For this review, take the finished solid that the model builds, in its own axes (mm). Face numbers are marked on the shaded views. A direction names the side the tool comes from. Round coordinates to 2 decimals unless told otherwise and drop trailing zeros. Loops run counter-clockwise (first coordinate to the right, second up) from the corner with the lowest first, then second, coordinate; pieces in that order, holes last. Notation, with made-up numbers: M 42,72.5 L 76,72.5 A14 ccw 76,91.5 Z; hole C -35.5,72 d6. An arc over 180 degrees is marked long. One line per question, with ' | ' between items. Start each with the question number.
1) We need section B-B (y = -13.75). Give the boundary of the cut face in (x, z).
2) We need section C-C (z = 0). Give the boundary of the cut face in (x, y), and give its area (3 significant figures).
3) We need section D-D (x = -19). Give the boundary of the cut face in (y, z).
4) We need section A-A (x = 10.5). Give the boundary of the cut face in (y, z).
5) Mouldability with a two-part tool opening along X and no side actions: class the marked faces 1, 2 and 3 as pulls with the +X half, pulls with the -X half, needs draft (parallel to the pull), parting line crosses it, or undercut.
6) For probe 1 along X at (y, z) = (2.35, -32.5); probe 2 along Z at (x, y) = (46, 2.25); probe 3 along Z at (x, y) = (23, 1.95), list the stretches that pass through material, from the lowest coordinate up. Write a range as from..to.
7) For the marked faces 4, 5 and 6, list the 3-axis set-ups (+Z, -Z, +X, -X, +Y, -Y) from which the entire face can be reached by the end or side of a thin tool; tool diameter is ignored.
8) For pin 1 Ø4 at (x, z) = (20, 25.5) entering from -Y; pin 2 Ø6 at (y, z) = (-2.5, 17.5) entering from +X; pin 3 Ø4 at (x, z) = (-53.5, 6) entering from +Y; pin 4 Ø3 at (x, y) = (-11, 2.5) entering from -Z, all flat-tipped, find the tip position at first contact; note any pin that passes through.
```python
from build123d import *

# Parameters (mm, degrees)
TABLE_DEPTH                  = 4
PIEDS_START                  = 17
PIEDS_DEPTH                  = 17
ENL_V_MAT_EXTRU_3_DEPTH      = 93.240175629
ENL_V_MAT_EXTRU_3_DEPTH_BACK = 93.240175629
ESQUISSE5_W                  = 5
ESQUISSE5_H                  = 18
ENL_V_MAT_EXTRU_4_DEPTH      = 93.240175629
ENL_V_MAT_EXTRU_4_DEPTH_BACK = 93.240175629
ESQUISSE6_W                  = 43
ESQUISSE6_H                  = 18
CONG_1_R                     = 10
CHANFREIN1_SIZE              = 1
CONG_2_R                     = 3
ESQUISSE3_R                  = 1
ENL_V_MAT_EXTRU_5_DEPTH      = 18
ENL_V_MAT_EXTRU_6_DEPTH      = 93.240175629
ENL_V_MAT_EXTRU_6_DEPTH_BACK = 93.240175629
ESQUISSE4_R                  = 1
ESQUISSE8_W                  = 58
ESQUISSE8_H                  = 72
ENL_V_MAT_EXTRU_7_DEPTH      = 1
ENL_V_MAT_EXTRU_8_DEPTH      = 1
ENL_V_MAT_EXTRU_9_DEPTH      = 93.240175629
ENL_V_MAT_EXTRU_9_DEPTH_BACK = 93.240175629
ESQUISSE11_W                 = 53
ESQUISSE11_H                 = 1
CONG_3_R                     = 1
CONG_4_R                     = 3


with BuildPart() as part:
    # Esquisse1 → table (new body)
    with BuildSketch(Plane(origin=(0, 0, 0), x_dir=(1, 0, 0), z_dir=(0, 1, 0))):
        with BuildLine():
            Line((-49, -57.5), (49, -57.5))
            ThreePointArc((49, -57.5), (63.142135624, -51.642135624), (69, -37.5))
            Line((69, -37.5), (69, 37.5))
            ThreePointArc((69, 37.5), (63.142135624, 51.642135624), (49, 57.5))
            Line((49, 57.5), (-49, 57.5))
            ThreePointArc((-49, 57.5), (-63.142135624, 51.642135624), (-69, 37.5))
            Line((-69, 37.5), (-69, -37.5))
            ThreePointArc((-69, -37.5), (-63.142135624, -51.642135624), (-49, -57.5))
        make_face()
    extrude(amount=TABLE_DEPTH)

    # Esquisse2 → pieds (add)
    with BuildSketch(Plane.XZ.offset(PIEDS_START)):
        with BuildLine():
            Line((-49, 57.5), (-49, 37.5))
            Line((-49, 37.5), (-69, 37.5))
            ThreePointArc((-69, 37.5), (-63.142135624, 51.642135624), (-49, 57.5))
        make_face()
        with BuildLine():
            Line((-69, -37.5), (-49, -37.5))
            Line((-49, -37.5), (-49, -57.5))
            ThreePointArc((-49, -57.5), (-63.142135624, -51.642135624), (-69, -37.5))
        make_face()
        with BuildLine():
            Line((49, -57.5), (49, -37.5))
            Line((49, -37.5), (69, -37.5))
            ThreePointArc((69, -37.5), (63.142135624, -51.642135624), (49, -57.5))
        make_face()
        with BuildLine():
            Line((49, 57.5), (49, 37.5))
            Line((49, 37.5), (69, 37.5))
            ThreePointArc((69, 37.5), (63.142135624, 51.642135624), (49, 57.5))
        make_face()
    extrude(amount=-PIEDS_DEPTH)

    # Esquisse5 → Enlèv. mat.-Extru.3 (cut, two sides: drawn at the far end of the back side and taken through both)
    with BuildSketch(Plane(origin=(0, 4, 0), x_dir=(1, 0, 0), z_dir=(0, 1, 0)).offset(-ENL_V_MAT_EXTRU_3_DEPTH_BACK)):
        with Locations((-26.5, 48.5)):
            Rectangle(ESQUISSE5_W, ESQUISSE5_H)
        with Locations((21.5, 48.5)):
            Rectangle(ESQUISSE5_W, ESQUISSE5_H)
        with Locations((-26.5, -48.5)):
            Rectangle(ESQUISSE5_W, ESQUISSE5_H)
        with Locations((21.5, -48.5)):
            Rectangle(ESQUISSE5_W, ESQUISSE5_H)
    extrude(amount=ENL_V_MAT_EXTRU_3_DEPTH + ENL_V_MAT_EXTRU_3_DEPTH_BACK, mode=Mode.SUBTRACT)

    # Esquisse6 → Enlèv. mat.-Extru.4 (cut, two sides: drawn at the far end of the back side and taken through both)
    with BuildSketch(Plane(origin=(0, 4, 0), x_dir=(1, 0, 0), z_dir=(0, 1, 0)).offset(-ENL_V_MAT_EXTRU_4_DEPTH_BACK)):
        with Locations((-2.5, 48.5)):
            Rectangle(ESQUISSE6_W, ESQUISSE6_H)
        with Locations((-2.5, -48.5)):
            Rectangle(ESQUISSE6_W, ESQUISSE6_H)
    extrude(amount=ENL_V_MAT_EXTRU_4_DEPTH + ENL_V_MAT_EXTRU_4_DEPTH_BACK, mode=Mode.SUBTRACT)

    # Congé1
    cong_1_edges = [part.edges().sort_by_distance(p)[0] for p in [
        (24, 2, 57.5),
        (-29, 2, -57.5),
        (24, 2, -57.5),
        (-29, 2, 57.5),
    ]]
    fillet(cong_1_edges, radius=CONG_1_R)

    # Chanfrein1
    chanfrein1_edges = [part.edges().sort_by_distance(p)[0] for p in [
        (59, -17, -37.5),
        (49, -17, -47.5),
        (63.142135624, -17, -51.642135624),
        (-49, -17, -47.5),
        (-59, -17, -37.5),
        (-63.142135624, -17, -51.642135624),
        (-59, -17, 37.5),
        (-49, -17, 47.5),
        (-63.142135624, -17, 51.642135624),
        (59, -17, 37.5),
        (63.142135624, -17, 51.642135624),
        (49, -17, 47.5),
    ]]
    chamfer(chanfrein1_edges, length=CHANFREIN1_SIZE)

    # Congé2
    cong_2_edges = [part.edges().sort_by_distance(p)[0] for p in [
        (49, -8, 37.5),
        (49, -8, -37.5),
        (-49, -8, -37.5),
        (-49, -8, 37.5),
    ]]
    fillet(cong_2_edges, radius=CONG_2_R)

    # Esquisse3 → Enlèv. mat.-Extru.5 (cut)
    with BuildSketch(Plane(origin=(0, 4, 0), x_dir=(1, 0, 0), z_dir=(0, 1, 0))):
        with Locations(Location((-10, -32.5, 0), (0, 0, 270))):
            Circle(ESQUISSE3_R)
        with Locations(Location((-61, -32.5, 0), (0, 0, 270))):
            Circle(ESQUISSE3_R)
        with Locations(Location((-61, 32.5, 0), (0, 0, 270))):
            Circle(ESQUISSE3_R)
        with Locations(Location((-10, 32.5, 0), (0, 0, 270))):
            Circle(ESQUISSE3_R)
    extrude(amount=-ENL_V_MAT_EXTRU_5_DEPTH, mode=Mode.SUBTRACT)

    # Esquisse4 → Enlèv. mat.-Extru.6 (cut, two sides: drawn at the far end of the back side and taken through both)
    with BuildSketch(Plane(origin=(0, 4, 0), x_dir=(1, 0, 0), z_dir=(0, 1, 0)).offset(-ENL_V_MAT_EXTRU_6_DEPTH_BACK)):
        with Locations(Location((2, -27, 0), (0, 0, 270))):
            Circle(ESQUISSE4_R)
        with Locations(Location((46, 17, 0), (0, 0, 270))):
            Circle(ESQUISSE4_R)
        with Locations(Location((23, 19, 0), (0, 0, 270))):
            Circle(ESQUISSE4_R)
    extrude(amount=ENL_V_MAT_EXTRU_6_DEPTH + ENL_V_MAT_EXTRU_6_DEPTH_BACK, mode=Mode.SUBTRACT)

    # Esquisse8 → Enlèv. mat.-Extru.7 (cut)
    with BuildSketch(Plane(origin=(0, 4, 0), x_dir=(1, 0, 0), z_dir=(0, 1, 0))):
        with Locations((-35.5, 0)):
            Rectangle(ESQUISSE8_W, ESQUISSE8_H)
    extrude(amount=-ENL_V_MAT_EXTRU_7_DEPTH, mode=Mode.SUBTRACT)

    # Esquisse10 → Enlèv. mat.-Extru.8 (cut)
    with BuildSketch(Plane(origin=(0, 4, 0), x_dir=(1, 0, 0), z_dir=(0, 1, 0))):
        Polygon((-2.5, -31.5), (50.207106781, -31.5), (60.5, -21.207106781), (60.5, 19.207106781), (48.207106781, 31.5), (7.792893219, 31.5), (-2.5, 21.207106781), align=None)
    extrude(amount=-ENL_V_MAT_EXTRU_8_DEPTH, mode=Mode.SUBTRACT)

    # Esquisse11 → Enlèv. mat.-Extru.9 (cut, two sides: drawn at the far end of the back side and taken through both)
    with BuildSketch(Plane(origin=(0, 4, 0), x_dir=(1, 0, 0), z_dir=(0, 1, 0)).offset(-ENL_V_MAT_EXTRU_9_DEPTH_BACK)):
        with Locations((-2.5, 39)):
            Rectangle(ESQUISSE11_W, ESQUISSE11_H)
        with Locations((-2.5, -39)):
            Rectangle(ESQUISSE11_W, ESQUISSE11_H)
    extrude(amount=ENL_V_MAT_EXTRU_9_DEPTH + ENL_V_MAT_EXTRU_9_DEPTH_BACK, mode=Mode.SUBTRACT)

    # Congé3
    cong_3_edges = [part.edges().sort_by_distance(p)[0] for p in [
        (24, 2, -38.5),
        (-29, 2, -38.5),
        (-29, 2, 38.5),
        (24, 2, 38.5),
    ]]
    fillet(cong_3_edges, radius=CONG_3_R)

    # Congé4
    # the kernel refuses this fillet: 3 mm, written as the material it takes off along each edge
    with BuildSketch(Plane(origin=(69, -24.858353806, 37.5), x_dir=(-1, 0, 0), z_dir=(0, 1, 0)), Plane(origin=(-69, -24.858353806, -37.5), x_dir=(1, 0, 0), z_dir=(0, 1, 0)), Plane(origin=(49, -24.858353806, -57.5), x_dir=(0, 0, 1), z_dir=(0, 1, 0)), Plane(origin=(-49, -24.858353806, 57.5), x_dir=(0, 0, -1), z_dir=(0, 1, 0))) as cong_4_piece_1:
        with BuildLine():
            CenterArc((3.266799469, 3), CONG_4_R, 169.835751378, 100.164248622)
            ThreePointArc((0.313881729, 3.529411765), (0.078624979, 1.771670761), (0, 0))
            Line((0, 0), (3.266799469, 0))
        make_face()
    extrude(amount=24.858353806, mode=Mode.SUBTRACT)
    with BuildSketch(Plane(origin=(-49, -24.858353806, -57.5), x_dir=(0, 0, 1), z_dir=(0, 1, 0)), Plane(origin=(-69, -24.858353806, 37.5), x_dir=(1, 0, 0), z_dir=(0, 1, 0)), Plane(origin=(69, -24.858353806, -37.5), x_dir=(-1, 0, 0), z_dir=(0, 1, 0)), Plane(origin=(49, -24.858353806, 57.5), x_dir=(0, 0, -1), z_dir=(0, 1, 0))) as cong_4_piece_2:
        with BuildLine():
            CenterArc((3.266799469, -3), CONG_4_R, 90, 100.164248622)
            ThreePointArc((0.313881729, -3.529411765), (0.078624979, -1.771670761), (0, 0))
            Line((0, 0), (3.266799469, 0))
        make_face()
    extrude(amount=24.858353806, mode=Mode.SUBTRACT)


solid = part.part
```
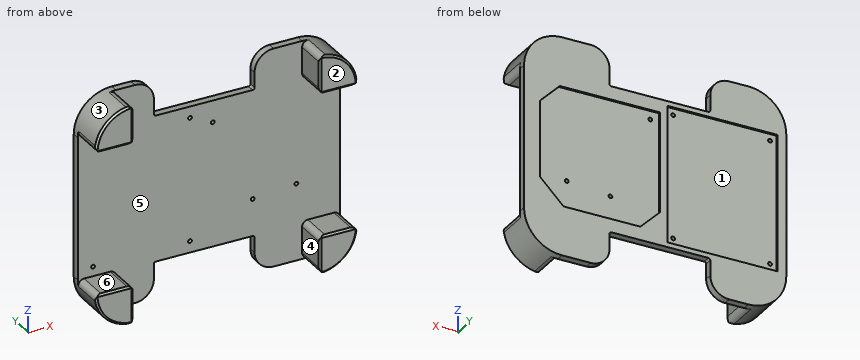
Answers below:
1) outline: M -68.69,-41.03 A20 ccw -52.53,-57.19 A3 ccw -49,-54.23 L -49,-40.5 A3 ccw -52,-37.5 L -65.73,-37.5 A3 ccw Z; M -68.69,41.03 A3 ccw -65.73,37.5 L -52,37.5 A3 ccw -49,40.5 L -49,54.23 A3 ccw -52.53,57.19 A20 ccw Z; M 49,-54.23 A3 ccw 52.53,-57.19 A20 ccw 68.69,-41.03 A3 ccw 65.73,-37.5 L 52,-37.5 A3 ccw 49,-40.5 Z; M 49,40.5 A3 ccw 52,37.5 L 65.73,37.5 A3 ccw 68.69,41.03 A20 ccw 52.53,57.19 A3 ccw 49,54.23 Z
2) outline: M -69,0 L 69,0 L 69,4 L 60.5,4 L 60.5,3 L -2.5,3 L -2.5,4 L -6.5,4 L -6.5,3 L -64.5,3 L -64.5,4 L -69,4 Z | area: 431 mm^2
3) outline: M 0,-38.5 L 4,-38.5 L 4,-36 L 3,-36 L 3,36 L 4,36 L 4,38.5 L 0,38.5 Z
4) outline: M 0,-38.5 L 4,-38.5 L 4,-31.5 L 3,-31.5 L 3,31.5 L 4,31.5 L 4,38.5 L 0,38.5 Z
5) face 1: undercut | face 2: needs draft | face 3: pulls with the -X half
6) probe 1: -69..-62, -60..-11, -9..69 | probe 2: -57.5..-18, -16..57.5 | probe 3: -38.5..-20, -18..38.5
7) face 4: +Z, -Z, -Y | face 5: -Y | face 6: +X, -X, -Y
8) pin 1: y = 0 | pin 2: x = 69 | pin 3: y = 3 | pin 4: z = -38.5
